Model file for the job. Use its own axes, mm. Face numbers are marked on the shaded views. A direction names the side the tool comes from. Round coordinates to 2 decimals unless told otherwise and drop trailing zeros. Order: outer loops, then holes, each group sorted by start corner. A loop starts at its lowest first (then second) coordinate and runs counter-clockwise, first axis right, second up. Notation, with made-up numbers: (-4.75, 78.5) - (27.25, 78.5) arc R28 cw to (27.25, 113.5) - close; hole circle Ø10 at (45, -12.5). An arc over 180 degrees is marked (long way). Write item = value, one per line. Start each with the question number.
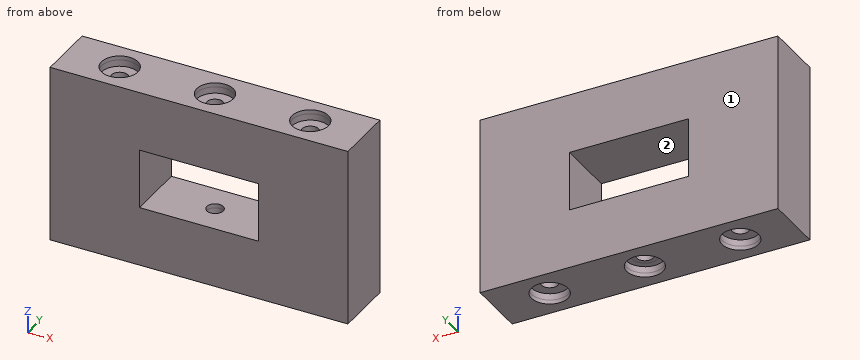
from build123d import *
from build123d.topology import SkipClean

# Parameters (mm, degrees)
SKETCH1_W                               = 100
SKETCH1_H                               = 60
BOSS_EXTRUDE1_DEPTH                     = 20
SKETCH2_W                               = 40
SKETCH2_H                               = 20
CUT_EXTRUDE1_DEPTH                      = 62.64414003
CBORE_FOR_M5_HEX_HEAD_BOLT1_D           = 5.5
CBORE_FOR_M5_HEX_HEAD_BOLT1_DEPTH       = 15
CBORE_FOR_M5_HEX_HEAD_BOLT1_CBORE_D     = 12.24
CBORE_FOR_M5_HEX_HEAD_BOLT1_CBORE_DEPTH = 3.58
CBORE_FOR_M5_HEX_HEAD_BOLT1_TIP         = 1.652366702
CBORE_FOR_M5_HEX_HEAD_BOLT2_D           = 5.5
CBORE_FOR_M5_HEX_HEAD_BOLT2_DEPTH       = 20
CBORE_FOR_M5_HEX_HEAD_BOLT2_CBORE_D     = 12.24
CBORE_FOR_M5_HEX_HEAD_BOLT2_CBORE_DEPTH = 3.58
CBORE_FOR_M5_HEX_HEAD_BOLT2_TIP         = 1.652366702
SHELL1_START                            = -48.6
SHELL1_2_OUTLINE_W                      = 17.2
SHELL1_2_OUTLINE_H                      = 17.2
SHELL1_2_DEPTH                          = 97.2
SHELL1_3_OUTLINE_W                      = 17.2
SHELL1_3_OUTLINE_H                      = 22.8
SHELL1_3_DEPTH                          = 27.2
SHELL1_START_2                          = 21.4
SHELL1_4_OUTLINE_W                      = 17.2
SHELL1_4_OUTLINE_H                      = 22.8
SHELL1_4_DEPTH                          = 27.2
SHELL1_START_3                          = -28.6
SHELL1_5_OUTLINE_R                      = 7.52
SHELL1_5_OUTLINE_R_2                    = 6.12
SHELL1_5_DEPTH                          = 3.58
SHELL1_START_4                          = -26.42
SHELL1_6_OUTLINE_R                      = 4.15
SHELL1_6_OUTLINE_R_2                    = 2.75
SHELL1_6_DEPTH                          = 15.02
SHELL1_7_OUTLINE_R                      = 6.12
SHELL1_7_OUTLINE_R_2                    = 4.15
SHELL1_7_DEPTH                          = 1.4


with BuildPart() as part:
    # Sketch1 → Boss-Extrude1 (new body)
    with BuildSketch(Plane(origin=(0, 0, 0), x_dir=(1, 0, 0), z_dir=(0, 1, 0))):
        Rectangle(SKETCH1_W, SKETCH1_H)
    extrude(amount=BOSS_EXTRUDE1_DEPTH)

    # Sketch2 → Cut-Extrude1 (cut, through all)
    with BuildSketch(Plane(origin=(0, 20, 0), x_dir=(1, 0, 0), z_dir=(0, 1, 0))):
        Rectangle(SKETCH2_W, SKETCH2_H)
    extrude(amount=-CUT_EXTRUDE1_DEPTH, mode=Mode.SUBTRACT)

    # CBORE for M5 Hex Head Bolt1
    with Locations(Plane.XY.offset(30)):
        with Locations((0, 10), (-32, 10), (32, 10)):
            CounterBoreHole(CBORE_FOR_M5_HEX_HEAD_BOLT1_D / 2, CBORE_FOR_M5_HEX_HEAD_BOLT1_CBORE_D / 2, CBORE_FOR_M5_HEX_HEAD_BOLT1_CBORE_DEPTH, depth=CBORE_FOR_M5_HEX_HEAD_BOLT1_DEPTH)
            with Locations((0, 0, -(CBORE_FOR_M5_HEX_HEAD_BOLT1_DEPTH + CBORE_FOR_M5_HEX_HEAD_BOLT1_TIP / 2))):  # 118° drill point
                Cone(0, CBORE_FOR_M5_HEX_HEAD_BOLT1_D / 2, CBORE_FOR_M5_HEX_HEAD_BOLT1_TIP, mode=Mode.SUBTRACT)

    # CBORE for M5 Hex Head Bolt2
    with Locations(Plane(origin=(0, 0, -30), x_dir=(-1, 0, 0), z_dir=(0, 0, -1))):
        with Locations((0, 10.04768743), (-31.999964467, 10), (31.999964467, 10)):
            CounterBoreHole(CBORE_FOR_M5_HEX_HEAD_BOLT2_D / 2, CBORE_FOR_M5_HEX_HEAD_BOLT2_CBORE_D / 2, CBORE_FOR_M5_HEX_HEAD_BOLT2_CBORE_DEPTH, depth=CBORE_FOR_M5_HEX_HEAD_BOLT2_DEPTH)
            with Locations((0, 0, -(CBORE_FOR_M5_HEX_HEAD_BOLT2_DEPTH + CBORE_FOR_M5_HEX_HEAD_BOLT2_TIP / 2))):  # 118° drill point
                Cone(0, CBORE_FOR_M5_HEX_HEAD_BOLT2_D / 2, CBORE_FOR_M5_HEX_HEAD_BOLT2_TIP, mode=Mode.SUBTRACT)

    # Shell1: read off the stored shape, not the designer's step
    # Shell1 outline → Shell1 (revolve, cut)
    with BuildSketch(Plane(origin=(-32, 10, 0), x_dir=(1, 0, 0), z_dir=(0, -1, 0))):
        Polygon((4.15, 14.207918111), (0, 11.714346542), (7.52, 11.714346542), (7.52, 25.02), (4.15, 25.02), align=None)
    revolve(axis=Axis((-32, 10, 0), (0, 0, 1)), mode=Mode.SUBTRACT)

    # Shell1 2 outline → Shell1 2 (cut)
    with BuildSketch(Plane.YZ.offset(SHELL1_START)):
        with Locations((10, -20)):
            Rectangle(SHELL1_2_OUTLINE_W, SHELL1_2_OUTLINE_H)
        with Locations((10, 20)):
            Rectangle(SHELL1_2_OUTLINE_W, SHELL1_2_OUTLINE_H)
    extrude(amount=SHELL1_2_DEPTH, mode=Mode.SUBTRACT)

    # Shell1 3 outline → Shell1 3 (cut)
    with BuildSketch(Plane.YZ.offset(SHELL1_START)):
        with Locations((10, 0)):
            Rectangle(SHELL1_3_OUTLINE_W, SHELL1_3_OUTLINE_H)
    extrude(amount=SHELL1_3_DEPTH, mode=Mode.SUBTRACT)

    # Shell1 4 outline → Shell1 4 (cut)
    with BuildSketch(Plane.YZ.offset(SHELL1_START_2)):
        with Locations((10, 0)):
            Rectangle(SHELL1_4_OUTLINE_W, SHELL1_4_OUTLINE_H)
    extrude(amount=SHELL1_4_DEPTH, mode=Mode.SUBTRACT)

    # Shell1 5 outline → Shell1 5 (add)
    # profile 1 of 3: a face of its own
    with SkipClean():  # the faces are left unmerged after this step: merging them gives an invalid solid
        with BuildSketch(Plane.XY.offset(SHELL1_START_3)):
            with Locations((0, 10.04768743)):
                Circle(SHELL1_5_OUTLINE_R)
            with Locations((0, 10.04768743)):
                Circle(SHELL1_5_OUTLINE_R_2, mode=Mode.SUBTRACT)
        # profile 2 of 3: a face of its own
        with BuildSketch(Plane.XY.offset(SHELL1_START_3)):
            with Locations((-31.999964467, 10)):
                Circle(SHELL1_5_OUTLINE_R)
            with Locations((-31.999964467, 10)):
                Circle(SHELL1_5_OUTLINE_R_2, mode=Mode.SUBTRACT)
        # profile 3 of 3: a face of its own
        with BuildSketch(Plane.XY.offset(SHELL1_START_3)):
            with Locations((31.999964467, 10)):
                Circle(SHELL1_5_OUTLINE_R)
            with Locations((31.999964467, 10)):
                Circle(SHELL1_5_OUTLINE_R_2, mode=Mode.SUBTRACT)
        extrude(amount=SHELL1_5_DEPTH)
    add(part.part.scale(1), mode=Mode.REPLACE)  # the faces are merged on a copy

    # Shell1 6 outline → Shell1 6 (add)
    with BuildSketch(Plane.XY.offset(SHELL1_START_4)):
        with Locations((0, 10.04768743)):
            Circle(SHELL1_6_OUTLINE_R)
        with Locations((0, 10.04768743)):
            Circle(SHELL1_6_OUTLINE_R_2, mode=Mode.SUBTRACT)
    extrude(amount=SHELL1_6_DEPTH)

    # Shell1 7 outline → Shell1 7 (add)
    with SkipClean():  # the faces are left unmerged after this step: merging them gives an invalid solid
        with BuildSketch(Plane.XY.offset(SHELL1_START_4)):
            with Locations((0, 10.04768743)):
                Circle(SHELL1_7_OUTLINE_R)
            with Locations((0, 10.04768743)):
                Circle(SHELL1_7_OUTLINE_R_2, mode=Mode.SUBTRACT)
        extrude(amount=SHELL1_7_DEPTH)

    # Shell1 8 outline → Shell1 8 (revolve)
    with SkipClean():  # the faces are left unmerged after this step: merging them gives an invalid solid
        with BuildSketch(Plane(origin=(32, 10, 0), x_dir=(1, 0, 0), z_dir=(0, -1, 0))):
            Polygon((0, 11.714346542), (4.15, 14.207918111), (4.15, 25.02), (7.52, 25.02), (7.52, 28.6), (6.12, 28.6), (6.12, 26.42), (2.75, 26.42), (2.75, 15), (0, 13.347633298), align=None)
        revolve(axis=Axis((32, 10, 0), (0, 0, 1)))

    # Shell1 9 outline → Shell1 9 (revolve)
    with SkipClean():  # the faces are left unmerged after this step: merging them gives an invalid solid
        with BuildSketch(Plane(origin=(-32, 10, 0), x_dir=(1, 0, 0), z_dir=(0, -1, 0))):
            Polygon((2.75, 26.42), (2.75, 15), (0, 13.347633298), (0, 11.714346542), (4.15, 14.207918111), (4.15, 25.02), (7.52, 25.02), (7.52, 28.6), (6.12, 28.6), (6.12, 26.42), align=None)
        revolve(axis=Axis((-32, 10, 0), (0, 0, 1)))

    # Shell1 10 outline → Shell1 10 (revolve)
    with SkipClean():  # the faces are left unmerged after this step: merging them gives an invalid solid
        with BuildSketch(Plane.XZ.offset(-10)):
            Polygon((2.75, 26.42), (2.75, 15), (0, 13.347633298), (0, 11.714346542), (4.15, 14.207918111), (4.15, 25.02), (7.52, 25.02), (7.52, 28.6), (6.12, 28.6), (6.12, 26.42), align=None)
        revolve(axis=Axis((0, 10, 0), (0, 0, 1)))

    # Shell1 11 outline → Shell1 11 (revolve)
    with BuildSketch(Plane(origin=(-31.999964467, 10, 0), x_dir=(1, 0, 0), z_dir=(0, -1, 0))):
        Polygon((0, -6.714346542), (0, -8.347633298), (2.75, -10), (2.75, -26.42), (6.12, -26.42), (6.12, -28.6), (7.52, -28.6), (7.52, -25.02), (4.15, -25.02), (4.15, -9.207918111), align=None)
    revolve(axis=Axis((-31.999964467, 10, 0), (0, 0, 1)))

    # Shell1 12 outline → Shell1 12 (revolve)
    with BuildSketch(Plane(origin=(31.999964467, 10, 0), x_dir=(1, 0, 0), z_dir=(0, -1, 0))):
        Polygon((2.75, -10), (2.75, -26.42), (6.12, -26.42), (6.12, -28.6), (7.52, -28.6), (7.52, -25.02), (4.15, -25.02), (4.15, -9.207918111), (0, -6.714346542), (0, -8.347633298), align=None)
    revolve(axis=Axis((31.999964467, 10, 0), (0, 0, 1)))


solid = part.part
Item 1: Saw through at C-C, the plane z = -23. Give the cut face in (x, y).
Item 2: Which spindle directions (+Z, -Z, +X, -X, +Y, -Y) get a long thin tool onto all of the face, cutting with end or side? Do the marked faces 1 and 2. Say none if no direction does.
Item 3: Saw through at B-B, the plane x = -41.5. Give the cut face in (y, z), then the cut area to 3 significant figures.
Item 4: Drop flat-ended pins along their axis: pin 1 (4.5 mm diameter, centred on x = 0, y = 10, fed in from -Z); pin 2 (10 mm diameter, centred on x = -32, y = 10, fed in from +Z); pin 3 (6 mm diameter, centred on x = 29, y = 12, fed in from -Z); pin 4 (4.5 mm diameter, centred on x = -32, y = 10, fed in from +Z). Give the stop position or say it passes through.
Item 5: Probe L1, parallel to Y at x = 32, z = 27.1; L2, parallel to Z at x = 4.5, y = 11; L3, parallel to Z at x = -19.5, y = 3.5. List the from-to ranges inside material, lowest first.
Item 6: Saw through at A-A, the plane x = -19. Give the cut face in (y, z).
Check sheet entries:
q1.outline = (-50, 0) - (50, 0) - (50, 20) - (-50, 20) - close; circle Ø8.3 at (-32, 10); circle Ø8.3 at (0, 10.05); circle Ø8.3 at (32, 10); hole (-48.6, 1.4) - (48.6, 1.4) - (48.6, 18.6) - (-48.6, 18.6) - close; hole circle Ø5.5 at (-32, 10); hole circle Ø5.5 at (0, 10.05); hole circle Ø5.5 at (32, 10)
q2.face_1 = +Z, -Z, +X, -X, +Y
q2.face_2 = +Y, -Y
q3.outline = (0, -30) - (20, -30) - (20, 30) - (0, 30) - close; hole (1.4, -28.6) - (18.6, -28.6) - (18.6, 28.6) - (1.4, 28.6) - close
q3.area = 216 mm2
q4.pin_1 = 10
q4.pin_2 = 26.42
q4.pin_3 = -30
q4.pin_4 = 14.7
q5.L1 = 0 to 1.4, 2.48 to 3.88, 16.12 to 17.52, 18.6 to 20
q5.L2 = -26.42 to -25.02, -11.4 to -10, 10 to 11.4, 25.02 to 26.42
q5.L3 = -30 to -28.6, -11.4 to -10, 10 to 11.4, 28.6 to 30
q6.outline = (0, -30) - (20, -30) - (20, -10) - (0, -10) - close; (0, 10) - (20, 10) - (20, 30) - (0, 30) - close; hole (1.4, -28.6) - (18.6, -28.6) - (18.6, -11.4) - (1.4, -11.4) - close; hole (1.4, 11.4) - (18.6, 11.4) - (18.6, 28.6) - (1.4, 28.6) - close
